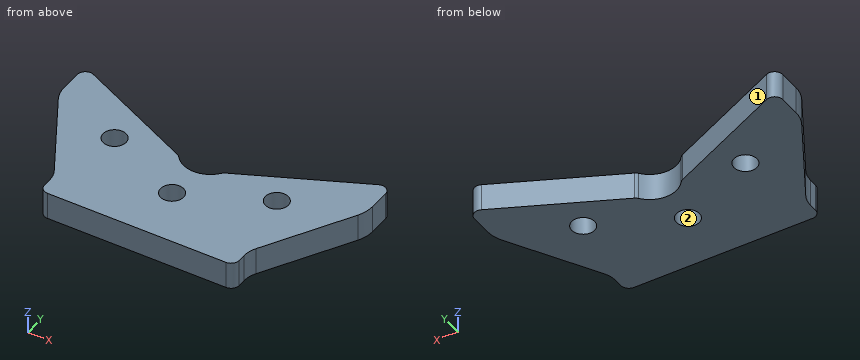
from build123d import *

# Parameters (mm, degrees)
EXTRUDE1_DEPTH         = 10
M10_GEVINDHULLER_D     = 8.5
M10_GEVINDHULLER_DEPTH = 22
M10_GEVINDHULLER_TIP   = 2.553657631


with BuildPart() as part:
    # Sketch1 → Extrude1 (new body)
    with BuildSketch(Plane.XY):
        with BuildLine():
            Line((-37.339745962, 10.947441117), (-55.392304845, 42.215390309))
            ThreePointArc((-55.392304845, 42.215390309), (-56.591109915, 45.109561768), (-57, 48.215390309))
            Line((-57, 48.215390309), (-57, 56))
            ThreePointArc((-57, 56), (-55.611898825, 58.530174337), (-52.732145215, 58.718923361))
            Line((-52.732145215, 58.718923361), (-8.939617358, 38.298132251))
            ThreePointArc((-8.939617358, 38.298132251), (-8.345295598, 37.931292757), (-7.851901649, 37.436973043))
            ThreePointArc((-7.851901649, 37.436973043), (0, 33.629520217), (7.851901649, 37.436973043))
            ThreePointArc((7.851901649, 37.436973043), (8.345295598, 37.931292757), (8.939617358, 38.298132251))
            Line((8.939617358, 38.298132251), (52.732145215, 58.718923361))
            ThreePointArc((52.732145215, 58.718923361), (55.611898825, 58.530174337), (57, 56))
            Line((57, 56), (57, 48.215390309))
            ThreePointArc((57, 48.215390309), (56.591109915, 45.109561768), (55.392304845, 42.215390309))
            Line((55.392304845, 42.215390309), (37.339745962, 10.947441117))
            ThreePointArc((37.339745962, 10.947441117), (36.340741737, 8.535631568), (36, 5.947441117))
            Line((36, 5.947441117), (36, 3))
            ThreePointArc((36, 3), (35.121320344, 0.878679656), (33, 0))
            Line((33, 0), (0, 0))
            Line((0, 0), (-33, 0))
            ThreePointArc((-33, 0), (-35.121320344, 0.878679656), (-36, 3))
            Line((-36, 3), (-36, 5.947441117))
            ThreePointArc((-36, 5.947441117), (-36.340741737, 8.535631568), (-37.339745962, 10.947441117))
        make_face()
    extrude(amount=EXTRUDE1_DEPTH)

    # M10 gevindhuller
    with Locations(Plane.XY.offset(10)):
        with Locations((-30, 34.878214934), (30, 34.878214934), (0, 20.878214934)):
            Hole(M10_GEVINDHULLER_D / 2, depth=M10_GEVINDHULLER_DEPTH)
            with Locations((0, 0, -(M10_GEVINDHULLER_DEPTH + M10_GEVINDHULLER_TIP / 2))):  # 118° drill point
                Cone(0, M10_GEVINDHULLER_D / 2, M10_GEVINDHULLER_TIP, mode=Mode.SUBTRACT)


solid = part.part
Here's how the part is built. I have some questions about the finished solid (model axes, mm). Face numbers are marked on the shaded views. A direction names the side the tool comes from. Give positions to 0.01 mm unless a question says otherwise; leave off trailing zeros. Order: outer loops, then holes, each group sorted by start corner. A loop starts at its lowest first (then second) coordinate and runs counter-clockwise, first axis right, second up. Notation, with made-up numbers: (61, 6) -> (112, 6) arc R15 ccw to (112, 35) -> close; hole circle Ø4 at (54.25, 9.5). An arc over 180 degrees is marked (long way). Use a Markdown table: item, result. Add a question column.
Item 1: For the marked faces 1 and 2, which set-ups out of +Z, -Z, +X, -X, +Y, -Y let a thin tool reach every point of the face, with its end or its side?
Item 2: Will these pins go through, and if not, where does the flat tip stop? pin 1 (0.9 mm diameter, centred on y = 4.5, z = 5.5, fed in from -X); pin 2 (4 mm diameter, centred on y = 38.5, z = 4, fed in from +X); pin 3 (1 mm diameter, centred on y = 39.5, z = 7.5, fed in from -X).
Item 3: Imagine slicing it at D-D on x = 17. Please give me the cut outline in (y, z), plus the area to 3 significant figures.
Item 4: Imagine slicing it at A-A on x = 0. Please give me the cut outline in (y, z), plus the area to 3 significant figures.
Item 5: Imagine slicing it at B-B on y = 44. Please give me the cut outline in (x, z), plus the area to 3 significant figures.
Item 6: Imagine slicing it at C-C on z = 3. Please give me the cut outline in (x, y), plus the area to 3 significant figures.
Item 7: I need wall thicknesses on line 1 (X direction, y = 36.5, z = 8.5); line 2 (X direction, y = 32.5, z = 6.75); line 3 (X direction, y = 4, z = 5.5). Which ranges of each line are inside material? Lowest first, please.
Data:
| question | item | result |
|---|---|---|
| 1 | face 1 | +Z, -Z, +Y |
| 1 | face 2 | +Z, -Z |
| 2 | pin 1 | stops at x = -36 |
| 2 | pin 2 | stops at x = 54.4 |
| 2 | pin 3 | stops at x = -54.11 |
| 3 | outline | (0, 0) -> (42.06, 0) -> (42.06, 10) -> (0, 10) -> close |
| 3 | area | 421 mm² |
| 4 | outline | (0, 0) -> (16.63, 0) -> (16.63, 10) -> (0, 10) -> close; (25.13, 0) -> (33.63, 0) -> (33.63, 10) -> (25.13, 10) -> close |
| 4 | area | 251 mm² |
| 5 | outline | (-56.24, 0) -> (-21.17, 0) -> (-21.17, 10) -> (-56.24, 10) -> close; (21.17, 0) -> (56.24, 0) -> (56.24, 10) -> (21.17, 10) -> close |
| 5 | area | 701 mm² |
| 6 | outline | (-57, 48.22) arc R12 ccw to (-55.39, 42.22) -> (-37.34, 10.95) arc R10 cw to (-36, 5.95) -> (-36, 3) arc R3 ccw to (-33, 0) -> (33, 0) arc R3 ccw to (36, 3) -> (36, 5.95) arc R10 cw to (37.34, 10.95) -> (55.39, 42.22) arc R12 ccw to (57, 48.22) -> (57, 56) arc R3 ccw to (52.73, 58.72) -> (8.94, 38.3) arc R3 ccw to (7.85, 37.44) arc R10 cw to (-7.85, 37.44) arc R3 ccw to (-8.94, 38.3) -> (-52.73, 58.72) arc R3 ccw to (-57, 56) -> close; hole circle Ø8.5 at (-30, 34.88); hole circle Ø8.5 at (0, 20.88); hole circle Ø8.5 at (30, 34.88) |
| 6 | area | 4,080 mm² |
| 7 | line 1 | x = -52.09 to -33.93, -26.07 to -7.01, 7.01 to 26.07, 33.93 to 52.09 |
| 7 | line 2 | x = -49.78 to -33.52, -26.48 to 26.48, 33.52 to 49.78 |
| 7 | line 3 | x = -36 to 36 |
